from build123d import *

# Parameters (mm, degrees)
SKETCH1_W           = 42
SKETCH1_H           = 42
BOSS_EXTRUDE1_DEPTH = 40
CHAMFER2_SIZE       = 3
SKETCH2_R           = 11
BOSS_EXTRUDE2_DEPTH = 2
BOSS_EXTRUDE3_DEPTH = 22
CHAMFER3_SIZE       = 1


with BuildPart() as part:
    # Sketch1 → Boss-Extrude1 (new body)
    with BuildSketch(Plane(origin=(0, 0, 0), x_dir=(1, 0, 0), z_dir=(0, 1, 0))):
        Rectangle(SKETCH1_W, SKETCH1_H)
    extrude(amount=BOSS_EXTRUDE1_DEPTH)

    # Chamfer2
    chamfer2_edges = [part.edges().sort_by_distance(p)[0] for p in [
        (21, 20, 21),
        (-21, 20, 21),
        (-21, 20, -21),
        (21, 20, -21),
    ]]
    chamfer(chamfer2_edges, length=CHAMFER2_SIZE)

    # Sketch2 → Boss-Extrude2 (add)
    with BuildSketch(Plane(origin=(0, 40, 0), x_dir=(1, 0, 0), z_dir=(0, 1, 0))):
        Circle(SKETCH2_R)
    extrude(amount=BOSS_EXTRUDE2_DEPTH)

    # Sketch3 → Boss-Extrude3 (add)
    with BuildSketch(Plane(origin=(0, 42, 0), x_dir=(1, 0, 0), z_dir=(0, 1, 0))):
        with BuildLine():
            Line((2.5, 1.658312395), (2.5, -1.658312395))
            ThreePointArc((2.5, -1.658312395), (-3, 0), (2.5, 1.658312395))
        make_face()
    extrude(amount=BOSS_EXTRUDE3_DEPTH)

    # Chamfer3
    chamfer3_edges = [part.edges().sort_by_distance(p)[0] for p in [
        (-11, 42, 0),
    ]]
    chamfer(chamfer3_edges, length=CHAMFER3_SIZE)


solid = part.part
Check sheet for the modelled part. Datum: model origin and axes. Units: mm. A direction names the side the tool comes from. Coordinates: 2 decimals unless noted, no trailing zeros. Loops run counter-clockwise (first coordinate to the right, second up) from the corner with the lowest first, then second, coordinate; pieces in that order, holes last. Notation, with made-up numbers: (67.25, 67.5) -> (84.25, 67.5) arc R20 cw to (84.25, 76.5) -> close; hole circle Ø4 at (-33, 16.25). An arc over 180 degrees is marked (long way). Write item = value, one per line. Start each with the question number.
1. Section check A-A on x = 0. Record the cut outline in (y, z), then the cut area to 4 significant figures.
2. Material ranges on line 1 (Y direction, x = 4.5, z = 18.5); line 2 (Y direction, x = 1, z = 3); line 3 (X direction, y = 42.5, z = 2), recorded low to high.
3. Tool access check on faces 1 (the flat face through (2.5, 53, 0)), 2 (the flat face through (2.1, 42, -2.4)), 3 (the flat face through (21, 20, 0)). Record the directions out of +Z, -Z, +X, -X, +Y, -Y that give a thin tool (end or side, any length) a straight path to the whole face; none if there is none.
4. Depth check by flat-ended pin: P1, Ø3.5, axis at y = 58, z = -0.5, coming from the +X side; P2, Ø4, axis at y = 52, z = 4.5, coming from the +X side; P3, Ø5, axis at x = -14.5, z = -2.5, coming from the +Y side. Enter the tip coordinate at first touch or a pass-through.
5. Section check B-B on y = 43.5. Record the cut outline in (x, z), then the cut area to 3 significant figures.
Responses:
q1.outline = (0, -21) -> (40, -21) -> (40, -11) -> (41, -11) -> (42, -10) -> (42, -3) -> (64, -3) -> (64, 3) -> (42, 3) -> (42, 10) -> (41, 11) -> (40, 11) -> (40, 21) -> (0, 21) -> close
q1.area = 1,855 mm2
q2.line_1 = 0 to 40
q2.line_2 = 0 to 42
q2.line_3 = -2.24 to 2.24
q3.face_1 = +Z, -Z, +X, +Y
q3.face_2 = +Y
q3.face_3 = +Z, -Z, +X, +Y, -Y
q4.P1 = 2.5
q4.P2 = 1.66
q4.P3 = 40
q5.outline = (2.5, -1.66) -> (2.5, 1.66) arc R3 ccw (long way) to start
q5.area = 27.1 mm2
